Autodesk Fusion 360 part; units mm, degrees
sketch "Sketch1" plane through (0, 0, 0) normal (0, 1, 0) x (1, 0, 0)
  line L0 (50, 5) -> (50, -5)
  line L1 (50, -5) -> (-50, -5)
  line L2 (-50, -5) -> (-50, 5)
  line L3 (0, 5) -> (0, -20)
  line L4 (-50, 5) -> (-40, 5)
  line L5 (-40, 5) -> (0, 5)
  line L6 (40, 5) -> (50, 5)
  line L7 (0, 5) -> (40, 5)
  arc A0 (50, 5) -> (30, 45) centre (0, 5) ccw
  arc A1 (-30.0001, 45) -> (-50, 5) centre (0, 5) ccw
  arc A2 (40, 5) -> (24, 37) centre (0, 5) ccw
  arc A3 (-24, 37) -> (-40, 5) centre (0, 5) ccw
  arc A4 (-24, 37) -> (-30.0001, 45) centre (-27, 41) ccw
  line L8 (-24, 37) -> (24, 37)
  arc A5 (30, 45) -> (24, 37) centre (27, 41) ccw
  dimension "d1" = 10
  dimension "d2" = 100
  dimension "d6" = 10
  dimension "d7" = 10
  dimension "d8" = 50
  dimension "d9" = 50
  dimension "d10" = 10
extrude "Extrude1" add sketch "Sketch1" along normal blind 2 contours L5 L7 A2 A3 L8
extrude "Extrude2" add sketch "Sketch1" along normal blind 50 contours L0 L1 L3 L6 L7 | L6 A0 A2 A5 | L1 L2 L3 L4 L5 | L4 A1 A3 A4
extrude "Extrude3" cut 1 faces at (0, 50, 1.6667) along direction (0, -1, 0) blind 25
equation "d7 = d6"
equation "d10 = d6"
Work out the finished part from the listing and answer in its coordinate system (mm). A direction names the side the tool comes from. Round coordinates to 2 decimals unless told otherwise and drop trailing zeros. Write each loop counter-clockwise with the first axis right and the second up, starting at its lowest first coordinate (ties: lowest second). Pieces come first, ordered by that corner, then holes. Notation, with made-up numbers: (-17, -11) - (29, -11) arc R34 cw to (29, 22) - close; hole circle Ø1 at (-37, 20.5). An arc over 180 degrees is marked (long way). Return JSON: item names as keys, results as strings. Group by question number.
Q1. For faces 1 (the cylindrical face through (-35.89, 13.34, -22.66)), 2 (the flat face through (-1, 25, -4)), determine the directions among +Z, -Z, +X, -X, +Y, -Y from which every point of the face is accessible in a straight line to the end or side of a thin tool.
Q2. The part is cut by section D-D on z = -23.5. Write down the section's boundary in (x, y), then the cut area to 3 significant figures.
Q3. The part is cut by section A-A on z = -41. Write down the section's boundary in (x, y), then the cut area to 3 significant figures.
Q4. Each of these flat-tipped pins is pushed along its axis until it touches: pin 1 Ø1.5 at (y, z) = (19.5, -34.5) entering from +X; pin 2 Ø10 at (x, y) = (-29, 13.5) entering from -Z; pin 3 Ø8 at (x, z) = (16, -10) entering from +Y; pin 4 Ø3 at (x, y) = (8.5, 17) entering from -Z. Where does it stop, or does it pass through?
Q5. Find the intervals of material crossed by L1, parallel to X at y = 4.5, z = -19; L2, parallel to Z at x = -6.5, y = 10; L3, parallel to X at y = 4.25, z = -16.5, in increasing order.
Q6. The mould has two halves that part along X. Classify faces 3 (the cylindrical face through (35.66, 13.34, -23.12)), 4 (the flat face through (-50, 12, 0)), 5 (the cylindrical face through (44.575, 12.325, -27.65)): released by +X, released by -X, zero draft, split by the parting line, or undercut.
Q7. The part is cut by section B-B on y = 16.5. Write down the section's boundary in (x, z).
Q8. The part is cut by section C-C on x = 7.5. Write down the section's boundary in (y, z), then the cut area to 3 significant figures.
Solved:
{
 "1": {"face 1": "+Y", "face 2": "+Z, -Z, +X, -X, +Y"},
 "2": {"outline": "(-46.45, 0) - (46.45, 0) - (46.45, 25) - (35.46, 25) - (35.46, 2) - (-35.46, 2) - (-35.46, 25) - (-46.45, 25) - close", "area": "691 mm²"},
 "3": {"outline": "(-34.7, 0) - (-22, 0) - (-22, 25) - (-34.7, 25) - close; (22, 0) - (34.7, 0) - (34.7, 25) - (22, 25) - close", "area": "635 mm²"},
 "4": {"pin 1": "x = 40.91", "pin 2": "z = -46", "pin 3": "y = 2", "pin 4": "z = -5"},
 "5": {"L1": "-48 to -37.47, 37.47 to 48", "L2": "-5 to 5", "L3": "-48.66 to -38.31, 38.31 to 48.66"},
 "6": {"face 3": "undercut", "face 4": "released by -X", "face 5": "released by +X"},
 "7": {"outline": "(-50, -5) arc R50 ccw to (-30, -45) arc R5 ccw to (-24, -37) arc R40 cw to (-40, -5) - (40, -5) arc R40 cw to (24, -37) arc R5 ccw to (30, -45) arc R50 ccw to (50, -5) - (50, 5) - (-50, 5) - close"},
 "8": {"outline": "(0, -37) - (2, -37) - (2, -5) - (25, -5) - (25, 5) - (0, 5) - close", "area": "314 mm²"}
}
